The figure shows three views and two pictorial views of one solid part (mm, origin at its lowest corner). Answer the questions. A direction names the side the tool comes from. Coordinates: 2 decimals unless noted, no trailing zeros. Write each loop counter-clockwise with the first axis right and the second up, starting at its lowest first coordinate (ties: lowest second). Pieces come first, ordered by that corner, then holes. Notation, with made-up numbers: M 69,45.5 L 104,45.5 A25 cw 104,65.5 Z; hole C 60.25,34.25 d6. An arc over 180 degrees is marked long. Use CSV: the item, a comma, the result in double quotes.
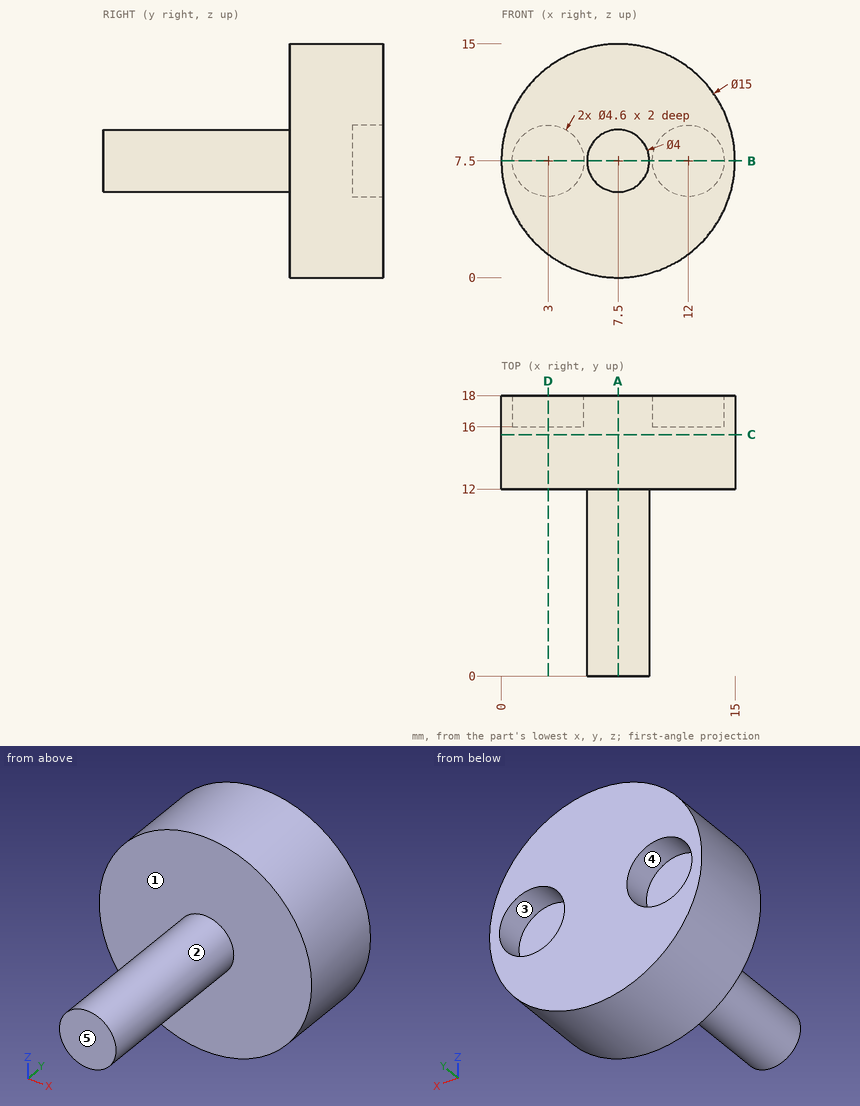
Item 1: For a pull along Z with two mould halves and no side action, classify the marked faces 1, 2 and 3 as released by +Z, released by -Z, zero draft, split by the parting line, or undercut.
Answer:
face 1,"zero draft"
face 2,"split by the parting line"
face 3,"undercut"
Item 2: Consider probe 1 along Y at (x, z) = (5, 10.5); probe 2 along Z at (x, y) = (3, 16.6); probe 3 along Z at (x, y) = (6.5, 7.5). Determine where each line is inside the solid, lowest interval first.
Answer:
probe 1,"y = 12 to 18"
probe 2,"z = 1.5 to 5.2, 9.8 to 13.5"
probe 3,"z = 5.77 to 9.23"
Item 3: Given pin 1 (5 mm diameter, centred on y = 2.5, z = 9, fed in from -X); pin 2 (1.5 mm diameter, centred on x = 11, z = 1.5, fed in from -Y); pin 3 (3 mm diameter, centred on x = 3, z = 7.5, fed in from +Y), each flat-ended and moving along its own axis, determine where each tip first touches the part or whether it passes through.
Answer:
pin 1,"stops at x = 5.5"
pin 2,"stops at y = 12"
pin 3,"stops at y = 16"
Item 4: The part is cut by section B-B (z = 7.5). Write down the section's boundary in (x, y).
Answer:
outline,"M 0,12 L 5.5,12 L 5.5,0 L 9.5,0 L 9.5,12 L 15,12 L 15,18 L 14.3,18 L 14.3,16 L 9.7,16 L 9.7,18 L 5.3,18 L 5.3,16 L 0.7,16 L 0.7,18 L 0,18 Z"
Item 5: The part is cut by section C-C (y = 15.5). Write down the section's boundary in (x, z).
Answer:
outline,"C 7.5,7.5 d15"
Item 6: The part is cut by section D-D (x = 3). Write down the section's boundary in (y, z), then the cut area to 3 significant figures.
Answer:
outline,"M 12,1.5 L 18,1.5 L 18,5.2 L 16,5.2 L 16,9.8 L 18,9.8 L 18,13.5 L 12,13.5 Z"
area,"62.8 mm2"
Item 7: The part is cut by section A-A (x = 7.5). Write down the section's boundary in (y, z).
Answer:
outline,"M 0,5.5 L 12,5.5 L 12,0 L 18,0 L 18,15 L 12,15 L 12,9.5 L 0,9.5 Z"
Item 8: A tool of negligible diameter and unlimited length cuts with its end or side. For the marked faces 4 and 5, from which of +Z, -Z, +X, -X, +Y, -Y can it reach the whole face along a straight path? Write none if from no direction.
Answer:
face 4,"+Y"
face 5,"+Z, -Z, +X, -X, -Y"
